Check sheet for the modelled part. Datum: model origin and axes. Units: mm. Face numbers are marked on the shaded views. A direction names the side the tool comes from. Round coordinates to 2 decimals unless told otherwise and drop trailing zeros. Loops run counter-clockwise (first coordinate to the right, second up) from the corner with the lowest first, then second, coordinate; pieces in that order, holes last. Notation, with made-up numbers: (0.5, 88) -> (34.5, 88) arc R21 ccw to (34.5, 121) -> close; hole circle Ø5 at (-18.5, -29). An arc over 180 degrees is marked (long way). Use one line per item in the form item = value. Start each with the question number.
(1) Draft check along Y on the marked faces 1, 2 and 3. Enter one of: released by +Y, released by -Y, zero draft, split by the parting line, or undercut.
(2) Set-up check for the marked faces 4, 5, 6 and 7: record each of +Z, -Z, +X, -X, +Y, -Y from which the full face is reachable in a straight line by a thin tool's end or side.
(3) Sectioned sample at C-C (y = 53.5). Record the cut outline in (x, z), and give its area (3 significant figures).
(4) Material ranges on probe 1 along Y at (x, z) = (-17, -10); probe 2 along Y at (x, z) = (-8, -31.5); probe 3 along Z at (x, y) = (10.5, 21.5), recorded low to high. Write a range as [from, to].
(5) Sectioned sample at B-B (x = 19). Record the cut outline in (y, z).
(6) Sectioned sample at D-D (x = -51.5). Record the cut outline in (y, z).
(7) Go/stop test with flat-tipped pins: pin 1 (4 mm diameter, centred on x = 9.5, z = 2.5, fed in from -Y); pin 2 (6 mm diameter, centred on x = -18, z = -8.5, fed in from -Y); pin 3 (16.5 mm diameter, centred on x = -17, y = -64.5, fed in from +Z); pin 4 (3 mm diameter, centred on x = 17, y = -7.5, fed in from +Z). Record where each tip stops, or that it passes through.
(8) Sectioned sample at A-A (z = -33). Record the cut outline in (x, y).
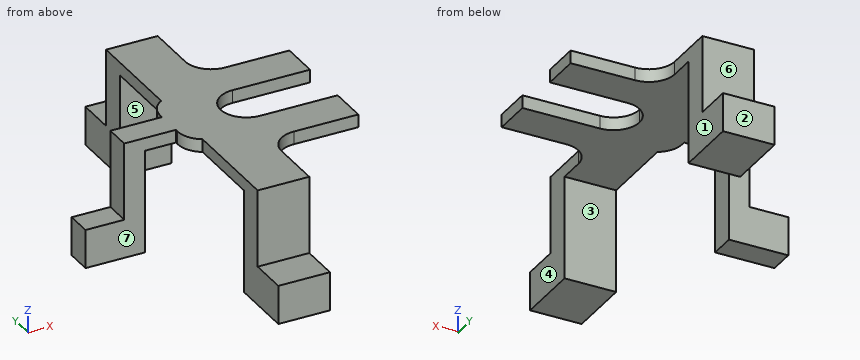
from build123d import *

# Parameters (mm, degrees)
SKETCH_1_W          = 60
SKETCH_1_H          = 30
EXTRUDE_1_DEPTH     = 5
SKETCH_2_W          = 7.4
SKETCH_2_H          = 1.2
SKETCH_2_W_2        = 7
SKETCH_2_H_2        = 0.8
CUT_EXTRUDE_1_DEPTH = 10
SKETCH_3_W          = 40.4
SKETCH_3_H          = 20.4
SKETCH_3_W_2        = 40
SKETCH_3_H_2        = 20
CUT_EXTRUDE_2_DEPTH = 10
SKETCH_5_W          = 20
SKETCH_5_H          = 40
SKETCH_5_H_2        = 10
EXTRUDE_2_DEPTH     = 5
SKETCH_6_W          = 20
SKETCH_6_H          = 10
SKETCH_6_W_2        = 8
EXTRUDE_3_DEPTH     = 40
SKETCH_7_W          = 20
SKETCH_7_H          = 15
SKETCH_7_W_2        = 15
SKETCH_7_H_2        = 10
EXTRUDE_4_DEPTH     = 15
SKETCH_8_W          = 54.931929912
SKETCH_8_H          = 24.682509144
EXTRUDE_5_DEPTH     = 5
SKETCH_9_W          = 40
SKETCH_9_H          = 20
CUT_EXTRUDE_3_DEPTH = 5
SKETCH_10_W         = 35
SKETCH_10_H         = 10
EXTRUDE_6_DEPTH     = 5
FILLET_2_R          = 10
FILLET_3_R          = 10


# Some blends are built 0.0001 mm under size
with BuildPart() as part:
    # 草图1 → 凸台-拉伸1 (new body)
    with BuildSketch(Plane.XY):
        Rectangle(SKETCH_1_W, SKETCH_1_H)
        Polygon((20, 0.4), (20, 10), (-20, 10), (-20, 0.4), (-27, 0.4), (-27, -0.4), (-20, -0.4), (-20, -10), (20, -10), (20, -0.4), (27, -0.4), (27, 0.4), align=None, mode=Mode.SUBTRACT)
    extrude(amount=EXTRUDE_1_DEPTH)

    # 草图2 → 切除-拉伸1 (cut)
    # profile 1 of 2: a face of its own
    with BuildSketch(Plane.XY.offset(5)):
        with Locations((-23.5, 0)):
            Rectangle(SKETCH_2_W, SKETCH_2_H)
        with Locations((-23.5, 0)):
            Rectangle(SKETCH_2_W_2, SKETCH_2_H_2, mode=Mode.SUBTRACT)
    # profile 2 of 2: a face of its own
    with BuildSketch(Plane.XY.offset(5)):
        with Locations((23.5, 0)):
            Rectangle(SKETCH_2_W, SKETCH_2_H)
        with Locations((23.5, 0)):
            Rectangle(SKETCH_2_W_2, SKETCH_2_H_2, mode=Mode.SUBTRACT)
    extrude(amount=-CUT_EXTRUDE_1_DEPTH, mode=Mode.SUBTRACT)

    # 草图3 → 切除-拉伸2 (cut)
    with BuildSketch(Plane.XY.offset(5)):
        Rectangle(SKETCH_3_W, SKETCH_3_H)
        Rectangle(SKETCH_3_W_2, SKETCH_3_H_2, mode=Mode.SUBTRACT)
    extrude(amount=-CUT_EXTRUDE_2_DEPTH, mode=Mode.SUBTRACT)

    # 草图5 → 凸台-拉伸2 (add)
    with BuildSketch(Plane(origin=(0, 0, 0), x_dir=(-1, 0, 0), z_dir=(0, 0, -1))):
        with Locations((15, 35)):
            Rectangle(SKETCH_5_W, SKETCH_5_H)
        with Locations((15, -35)):
            Rectangle(SKETCH_5_W, SKETCH_5_H)
        with Locations((40, 0)):
            Rectangle(SKETCH_5_W, SKETCH_5_H_2)
    extrude(amount=-EXTRUDE_2_DEPTH)

    # 草图6 → 凸台-拉伸3 (add)
    with BuildSketch(Plane(origin=(0, 0, 0), x_dir=(-1, 0, 0), z_dir=(0, 0, -1))):
        with Locations((15, 50)):
            Rectangle(SKETCH_6_W, SKETCH_6_H)
        with Locations((15, -50)):
            Rectangle(SKETCH_6_W, SKETCH_6_H)
        with Locations((46, 0)):
            Rectangle(SKETCH_6_W_2, SKETCH_6_H)
    extrude(amount=EXTRUDE_3_DEPTH)

    # 草图7 → 凸台-拉伸4 (add)
    with BuildSketch(Plane(origin=(0, 0, -40), x_dir=(-1, 0, 0), z_dir=(0, 0, -1))):
        with Locations((15, 62.5)):
            Rectangle(SKETCH_7_W, SKETCH_7_H)
        with Locations((15, -62.5)):
            Rectangle(SKETCH_7_W, SKETCH_7_H)
        with Locations((57.5, 0)):
            Rectangle(SKETCH_7_W_2, SKETCH_7_H_2)
    extrude(amount=-EXTRUDE_4_DEPTH)

    # 草图8 → 凸台-拉伸5 (add)
    with BuildSketch(Plane.XY.offset(5)):
        Rectangle(SKETCH_8_W, SKETCH_8_H)
    extrude(amount=-EXTRUDE_5_DEPTH)

    # 草图9 → 切除-拉伸3 (cut)
    with BuildSketch(Plane.XY.offset(5)):
        with Locations((10, 0)):
            Rectangle(SKETCH_9_W, SKETCH_9_H)
    extrude(amount=-CUT_EXTRUDE_3_DEPTH, mode=Mode.SUBTRACT)

    # 草图10 → 凸台-拉伸6 (add)
    with BuildSketch(Plane.XY.offset(5)):
        with Locations((12.5, 20)):
            Rectangle(SKETCH_10_W, SKETCH_10_H)
        with Locations((12.5, -20)):
            Rectangle(SKETCH_10_W, SKETCH_10_H)
    extrude(amount=-EXTRUDE_6_DEPTH)

    # 圆角2
    fillet_2_edges = [part.edges().sort_by_distance(p)[0] for p in [
        (-10, -10, 2.5),
        (-10, 10, 2.5),
        (-5, -25, 2.5),
        (-5, 25, 2.5),
    ]]
    fillet(fillet_2_edges, radius=FILLET_2_R - 0.0001)  # a hair under: the kernel refuses the full size

    # 圆角3
    # the kernel refuses this fillet: 10 mm, written as the material it takes off along each edge
    with BuildSketch(Plane(origin=(-30, -15, -21.650635095), x_dir=(0, 1, 0), z_dir=(0, 0, 1))) as fillet_3_piece_1:
        with BuildLine():
            CenterArc((8.660254038, -10), FILLET_3_R, 90, 60)
            Line((0, -5), (-0.173205081, -4.9))
            ThreePointArc((-0.173205081, -4.9), (-0.2, -2.5), (-0.2, 0))
            Line((-0.2, 0), (0, 0.2))
            Line((0, 0.2), (8.660254038, 0.2))
            Line((8.660254038, 0.2), (8.660254038, 0))
        make_face()
    extrude(amount=48.301270189, mode=Mode.SUBTRACT)
    with BuildSketch(Plane(origin=(-30, 15, -21.650635095), x_dir=(1, 0, 0), z_dir=(0, 0, 1))) as fillet_3_piece_2:
        with BuildLine():
            CenterArc((10, -8.660254038), FILLET_3_R, 120, 60)
            Line((0, -8.660254038), (-0.2, -8.660254038))
            Line((-0.2, -8.660254038), (-0.2, 0))
            Line((-0.2, 0), (0, 0.2))
            ThreePointArc((0, 0.2), (2.5, 0.2), (4.9, 0.173205081))
            Line((4.9, 0.173205081), (5, 0))
        make_face()
    extrude(amount=48.301270189, mode=Mode.SUBTRACT)


solid = part.part
Checks:
q1.face_1 = zero draft
q1.face_2 = released by +Y
q1.face_3 = undercut
q2.face_4 = +Z, -Z, +X, -Y
q2.face_5 = -Z, +X, -X
q2.face_6 = +Z, +X, -X, +Y
q2.face_7 = +Z, -Z, -X, -Y
q3.outline = (-25, -40) -> (-5, -40) -> (-5, 5) -> (-25, 5) -> close
q3.area = 900 mm2
q4.probe_1 = [-55, -45], [45, 55]
q4.probe_2 = [-70, -45], [45, 70]
q4.probe_3 = [0, 5]
q5.outline = (-25, 0) -> (-10, 0) -> (-10, 5) -> (-25, 5) -> close; (10, 0) -> (25, 0) -> (25, 5) -> (10, 5) -> close
q6.outline = (-5, -40) -> (5, -40) -> (5, -25) -> (-5, -25) -> close
q7.pin_1 = -25
q7.pin_2 = -55
q7.pin_3 = -25
q7.pin_4 = through
q8.outline = (-65, -5) -> (-42, -5) -> (-42, 5) -> (-65, 5) -> close; (-25, -70) -> (-5, -70) -> (-5, -45) -> (-25, -45) -> close; (-25, 45) -> (-5, 45) -> (-5, 70) -> (-25, 70) -> close
